Autodesk Inventor part; units mm, degrees
ref_plane "Work Plane1" through (-26.5, -2, 0) normal (-1, 0, 0) x (0, 0, 1)
ref_plane "YZ Plane" through (0, 0, 0) normal (1, 0, 0) x (0, 1, 0)
ref_plane "XZ Plane" through (0, 0, 0) normal (0, 1, 0) x (-1, 0, 0)
sketch "Sketch1" plane through (0, 0, 0) normal (0, 0, 1) x (1, 0, 0)
  line L0 (-25.25, 2.5) -> (25.25, 2.5)
  line L1 (25.25, 2.5) -> (25.25, -2.5)
  line L2 (25.25, -2.5) -> (-25.25, -2.5)
  line L3 (-25.25, -2.5) -> (-25.25, 2.5)
  circle A0 centre (-22.5, 1.3) radius 0.5
  circle A1 centre (-19.4, 1.3) radius 0.4
  circle A2 centre (-10.4, 1.3) radius 0.4
  circle A3 centre (-18, 1.3) radius 0.4
  circle A4 centre (-13.5, 1.3) radius 0.4
  circle A5 centre (-16.6, 1.3) radius 0.4
  circle A6 centre (-14.9, 1.3) radius 0.4
  circle A7 centre (-12.1, 1.3) radius 0.4
  circle A8 centre (-7.6, 1.3) radius 0.4
  circle A9 centre (-9, 1.3) radius 0.4
  line L4 (0, 0) -> (0, 2.997) construction
  line L5 (0, 0) -> (1.9732, 0) construction
  circle A10 centre (-4.5, 1.3) radius 0.5
  circle A11 centre (-1.5, 1.3) radius 0.4
  circle A12 centre (0, 1.3) radius 0.4
  circle A13 centre (1.5, 1.3) radius 0.4
  circle A14 centre (3, 1.3) radius 0.4
  circle A15 centre (4.5, 1.3) radius 0.4
  circle A16 centre (6, 1.3) radius 0.4
  circle A17 centre (7.5, 1.3) radius 0.4
  circle A18 centre (9, 1.3) radius 0.4
  circle A19 centre (10.5, 1.3) radius 0.4
  circle A20 centre (12, 1.3) radius 0.4
  circle A21 centre (13.5, 1.3) radius 0.4
  circle A22 centre (15, 1.3) radius 0.4
  circle A23 centre (18, 1.3) radius 0.625
  circle A24 centre (22.5, 1.3) radius 0.625
  line L6 (-22, 1.3) -> (-22, 2.5)
  line L7 (-23, 1.3) -> (-23, 2.5)
  line L8 (-19, 1.3) -> (-19, 2.5)
  line L9 (-19.8, 1.3) -> (-19.8, 2.5)
  line L10 (-17.6, 1.3) -> (-17.6, 2.5)
  line L11 (-18.4, 1.3) -> (-18.4, 2.5)
  line L12 (-16.2, 1.3) -> (-16.2, 2.5)
  line L13 (-17, 1.3) -> (-17, 2.5)
  line L14 (-14.5, 1.3) -> (-14.5, 2.5)
  line L15 (-15.3, 1.3) -> (-15.3, 2.5)
  line L16 (-13.1, 1.3) -> (-13.1, 2.5)
  line L17 (-13.9, 1.3) -> (-13.9, 2.5)
  line L18 (-11.7, 1.3) -> (-11.7, 2.5)
  line L19 (-12.5, 1.3) -> (-12.5, 2.5)
  line L20 (-10, 1.3) -> (-10, 2.5)
  line L21 (-10.8, 1.3) -> (-10.8, 2.5)
  line L22 (-8.6, 1.3) -> (-8.6, 2.5)
  line L23 (-9.4, 1.3) -> (-9.4, 2.5)
  line L24 (-7.2, 1.3) -> (-7.2, 2.5)
  line L25 (-8, 1.3) -> (-8, 2.5)
  line L26 (-4, 1.3) -> (-4, 2.5)
  line L27 (-5, 1.3) -> (-5, 2.5)
  line L28 (-1.1, 1.3) -> (-1.1, 2.5)
  line L29 (-1.9, 1.3) -> (-1.9, 2.5)
  line L30 (0.4, 1.3) -> (0.4, 2.5)
  line L31 (-0.4, 1.3) -> (-0.4, 2.5)
  line L32 (1.9, 1.3) -> (1.9, 2.5)
  line L33 (1.1, 1.3) -> (1.1, 2.5)
  line L34 (2.6, 1.3) -> (2.6, 2.5)
  line L35 (3.4, 1.3) -> (3.4, 2.5)
  line L36 (4.1, 1.3) -> (4.1, 2.5)
  line L37 (4.9, 1.3) -> (4.9, 2.5)
  line L38 (5.6, 1.3) -> (5.6, 2.5)
  line L39 (6.4, 1.3) -> (6.4, 2.5)
  line L40 (7.1, 1.3) -> (7.1, 2.5)
  line L41 (7.9, 1.3) -> (7.9, 2.5)
  line L42 (8.6, 1.3) -> (8.6, 2.5)
  line L43 (9.4, 1.3) -> (9.4, 2.5)
  line L44 (10.1, 1.3) -> (10.1, 2.5)
  line L45 (10.9, 1.3) -> (10.9, 2.5)
  line L46 (11.6, 1.3) -> (11.6, 2.5)
  line L47 (12.4, 1.3) -> (12.4, 2.5)
  line L48 (13.1, 1.3) -> (13.1, 2.5)
  line L49 (13.9, 1.3) -> (13.9, 2.5)
  line L50 (14.6, 1.3) -> (14.6, 2.5)
  line L51 (15.4, 1.3) -> (15.4, 2.5)
  line L52 (17.375, 1.3) -> (17.375, 2.5)
  line L53 (18.625, 1.3) -> (18.625, 2.5)
  line L54 (23.125, 1.3) -> (23.125, 2.5)
  line L55 (21.875, 1.3) -> (21.875, 2.5)
  circle A25 centre (22.5, -1.3) radius 0.625
  circle A26 centre (18, -1.3) radius 0.625
  circle A27 centre (15, -1.3) radius 0.4
  circle A28 centre (13.5, -1.3) radius 0.4
  circle A29 centre (12, -1.3) radius 0.4
  circle A30 centre (10.5, -1.3) radius 0.4
  circle A31 centre (9, -1.3) radius 0.4
  circle A32 centre (7.5, -1.3) radius 0.4
  circle A33 centre (6, -1.3) radius 0.4
  circle A34 centre (4.5, -1.3) radius 0.4
  circle A35 centre (3, -1.3) radius 0.4
  circle A36 centre (1.5, -1.3) radius 0.4
  circle A37 centre (0, -1.3) radius 0.4
  circle A38 centre (-1.5, -1.3) radius 0.4
  circle A39 centre (-7.5, -1.3) radius 0.4
  circle A40 centre (-9, -1.3) radius 0.4
  circle A41 centre (-10.5, -1.3) radius 0.4
  circle A42 centre (-12.6, -1.3) radius 0.4
  circle A43 centre (-14.4, -1.3) radius 0.4
  circle A44 centre (-16.5, -1.3) radius 0.4
  circle A45 centre (-18, -1.3) radius 0.4
  circle A46 centre (-19.5, -1.3) radius 0.4
  circle A47 centre (-21.6, -1.3) radius 0.4
  circle A48 centre (-23.4, -1.3) radius 0.4
  line L56 (23.125, -1.3) -> (23.125, -2.5)
  line L57 (21.875, -1.3) -> (21.875, -2.5)
  line L58 (18.625, -1.3) -> (18.625, -2.5)
  line L59 (17.375, -1.3) -> (17.375, -2.5)
  line L60 (15.4, -1.3) -> (15.4, -2.5)
  line L61 (14.6, -1.3) -> (14.6, -2.5)
  line L62 (13.9, -1.3) -> (13.9, -2.5)
  line L63 (13.1, -1.3) -> (13.1, -2.5)
  line L64 (12.4, -1.3) -> (12.4, -2.5)
  line L65 (11.6, -1.3) -> (11.6, -2.5)
  line L66 (10.9, -1.3) -> (10.9, -2.5)
  line L67 (10.1, -1.3) -> (10.1, -2.5)
  line L68 (9.4, -1.3) -> (9.4, -2.5)
  line L69 (8.6, -1.3) -> (8.6, -2.5)
  line L70 (7.9, -1.3) -> (7.9, -2.5)
  line L71 (7.1, -1.3) -> (7.1, -2.5)
  line L72 (6.4, -1.3) -> (6.4, -2.5)
  line L73 (5.6, -1.3) -> (5.6, -2.5)
  line L74 (4.9, -1.3) -> (4.9, -2.5)
  line L75 (4.1, -1.3) -> (4.1, -2.5)
  line L76 (3.4, -1.3) -> (3.4, -2.5)
  line L77 (2.6, -1.3) -> (2.6, -2.5)
  line L78 (1.9, -1.3) -> (1.9, -2.5)
  line L79 (1.1, -1.3) -> (1.1, -2.5)
  line L80 (0.4, -1.3) -> (0.4, -2.5)
  line L81 (-0.4, -1.3) -> (-0.4, -2.5)
  line L82 (-1.9, -1.3) -> (-1.9, -2.5)
  line L83 (-1.1, -1.3) -> (-1.1, -2.5)
  line L84 (-7.9, -1.3) -> (-7.9, -2.5)
  line L85 (-7.1, -1.3) -> (-7.1, -2.5)
  line L86 (-8.6, -1.3) -> (-8.6, -2.5)
  line L87 (-9.4, -1.3) -> (-9.4, -2.5)
  line L88 (-10.1, -1.3) -> (-10.1, -2.5)
  line L89 (-10.9, -1.3) -> (-10.9, -2.5)
  line L90 (-12.2, -1.3) -> (-12.2, -2.5)
  line L91 (-13, -1.3) -> (-13, -2.5)
  line L92 (-14, -1.3) -> (-14, -2.5)
  line L93 (-14.8, -1.3) -> (-14.8, -2.5)
  line L94 (-16.1, -1.3) -> (-16.1, -2.5)
  line L95 (-16.9, -1.3) -> (-16.9, -2.5)
  line L96 (-17.6, -1.3) -> (-17.6, -2.5)
  line L97 (-18.4, -1.3) -> (-18.4, -2.5)
  line L98 (-19.1, -1.3) -> (-19.1, -2.5)
  line L99 (-19.9, -1.3) -> (-19.9, -2.5)
  line L100 (-21.2, -1.3) -> (-21.2, -2.5)
  line L101 (-22, -1.3) -> (-22, -2.5)
  line L102 (-23, -1.3) -> (-23, -2.5)
  line L103 (-23.8, -1.3) -> (-23.8, -2.5)
  dimension "d0" = 50.5
  dimension "d1" = 5
  dimension "d3" = 1
  dimension "d4" = 2.75
  dimension "d5" = 0.8
  dimension "d6" = 0.8
  dimension "d7" = 0.8
  dimension "d8" = 0.8
  dimension "d9" = 0.8
  dimension "d10" = 0.8
  dimension "d11" = 0.8
  dimension "d12" = 0.8
  dimension "d13" = 0.8
  dimension "d14" = 3.1
  dimension "d15" = 1.4
  dimension "d16" = 1.4
  dimension "d17" = 1.4
  dimension "d18" = 1.4
  dimension "d19" = 1.7
  dimension "d20" = 1.4
  dimension "d21" = 1.4
  dimension "d22" = 1.7
  dimension "d23" = 1.2
  dimension "d24" = 1
  dimension "d25" = 3.1
  dimension "d26" = 0.8
  dimension "d27" = 0.8
  dimension "d28" = 0.8
  dimension "d29" = 0.8
  dimension "d30" = 0.8
  dimension "d31" = 0.8
  dimension "d32" = 0.8
  dimension "d33" = 0.8
  dimension "d34" = 0.8
  dimension "d35" = 0.8
  dimension "d36" = 0.8
  dimension "d37" = 0.8
  dimension "d38" = 3
  dimension "d39" = 1.5
  dimension "d40" = 1.5
  dimension "d41" = 1.5
  dimension "d42" = 1.5
  dimension "d43" = 1.5
  dimension "d44" = 1.5
  dimension "d45" = 1.5
  dimension "d46" = 1.5
  dimension "d47" = 1.5
  dimension "d48" = 1.5
  dimension "d49" = 1.5
  dimension "d50" = 1.25
  dimension "d51" = 1.25
  dimension "d52" = 3
  dimension "d53" = 4.5
  dimension "d121" = 1.25
  dimension "d122" = 1.25
  dimension "d125" = 0.8
  dimension "d126" = 0.8
  dimension "d127" = 0.8
  dimension "d128" = 0.8
  dimension "d129" = 0.8
  dimension "d130" = 0.8
  dimension "d131" = 0.8
  dimension "d132" = 0.8
  dimension "d133" = 0.8
extrude "Extrusion1" add sketch "Sketch1" along normal blind 2 contours L0 L7 A0 L6 L9 A1 L8 L11 A3 L10 L13 A5 L12 L15 A6 L14 L17 A4 L16 L19 A7 L18 L21 A2 L20 L23 A9 L22 L25 A8 L24 L27 A10 L26 L29 A11 L28 L31 A12 L30 L33 A13 L32 L34 A14 L35 L36 A15 L37 L38 A16 L39 L40 A17 L41 L42 A18 L43 L44 A19 L45 L46 A20 L47 L48 A21 L49 L50 A22 L51 L52 A23 L53 L55 A24 L54 L1 L2 L56 A25 L57 L58 A26 L59 L60 A27 L61 L62 A28 L63 L64 A29 L65 L66 A30 L67 L68 A31 L69 L70 A32 L71 L72 A33 L73 L74 A34 L75 L76 A35 L77 L78 A36 L79 L80 A37 L81 L83 A38 L82 L85 A39 L84 L86 A40 L87 L88 A41 L89 L90 A42 L91 L92 A43 L93 L94 A44 L95 L96 A45 L97 L98 A46 L99 L100 A47 L101 L102 A48 L103 L3
ref_plane "Work Plane1" through (-26.5, -2, 0) normal (-1, 0, 0) x (0, 0, 1)
sketch "Sketch12" plane through (0, 0, 0) normal (0, 0, -1) x (-1, 0, 0)
  arc A0 (-24.0126, -0.5173) -> (-23.9919, 1.0846) centre (-25.2704, 0.3) ccw
  arc A1 (-24.2504, 2) -> (-23.9919, 1.0846) centre (-22.5004, 2) ccw
  arc A2 (-24.0126, -0.5173) -> (-24.2331, -2) centre (-22.5004, -1.5) ccw
  line L0 (-24.2331, -2) -> (-25.0004, -2)
  line L1 (-25.0004, 2) -> (-24.2504, 2)
  line L2 (-25.0004, -2.1) -> (-24.0947, -2.1)
  arc A3 (-23.9286, -0.5716) -> (-23.8794, -2.5) centre (-22.5004, -1.5) ccw
  arc A4 (-23.9286, -0.5716) -> (-23.9067, 1.1369) centre (-25.2704, 0.3) ccw
  arc A5 (-24.1474, 2.1) -> (-23.9067, 1.1369) centre (-22.5004, 2) ccw
  line L3 (-24.1474, 2.1) -> (-25, 2.1)
  line L4 (-24.1474, 2.1) -> (-24.1474, 2.5)
  line L5 (-25.25, 2.5) -> (-23.125, 2.5)
  line L6 (-24.1474, 2.5) -> (-25.25, 2.5)
  line L7 (-23.125, -2.5) -> (-25.25, -2.5)
  line L8 (-25.25, 2.5) -> (-25.25, -2.5)
  line L9 (-25.25, -2.5) -> (-24.0947, -2.5)
  line L10 (-24.0947, -2.1) -> (-24.0947, -2.5)
  point P0 (0, 0)
  dimension "d188" = 0.1
extrude "Extrusion12" cut sketch "Sketch12" against normal blind 10
sketch "Sketch13" plane through (0, 0, 0) normal (0, 0, -1) x (-1, 0, 0)
  arc A0 (24.3834, 0.9639) -> (24.3834, -0.9639) centre (26.1358, 0) ccw
  arc A1 (24.3834, 0.9639) -> (24.6496, 2) centre (22.4996, 2) ccw
  arc A2 (24.6496, -2) -> (24.3834, -0.9639) centre (22.4996, -2) ccw
  line L0 (24.6496, -2) -> (25, -2)
  line L1 (24.9996, 2) -> (24.6496, 2)
  line L2 (24.6496, 2) -> (24.6496, 2.5)
  line L3 (23, 2.5) -> (25.25, 2.5)
  line L4 (24.6496, -2) -> (24.6496, -2.5)
  line L5 (25.25, -2.5) -> (23.8, -2.5)
  line L6 (24.6496, -2.5) -> (25.25, -2.5)
  line L7 (25.25, -2.5) -> (25.25, 2.5)
  line L8 (25.25, 2.5) -> (25.25, -2.5)
  line L9 (25.25, 2.5) -> (24.6496, 2.5)
  line L10 (25, -2.1) -> (24.5471, -2.1)
  arc A3 (24.5471, -2.1) -> (24.2958, -1.012) centre (22.4996, -2) ccw
  arc A4 (24.2958, 1.012) -> (24.2958, -1.012) centre (26.1358, 0) ccw
  arc A5 (24.2958, 1.012) -> (24.5471, 2.1) centre (22.4996, 2) ccw
  line L11 (24.5471, 2.1) -> (25, 2.1)
  line L12 (24.55, -2.6) -> (25.35, -2.6)
  line L13 (25.35, -2.6) -> (25.35, 2.6)
  line L14 (25.35, 2.6) -> (24.55, 2.6)
  line L15 (24.5471, -2.5) -> (24.6496, -2.5)
  line L16 (24.6496, 2.5) -> (24.5471, 2.5)
  line L17 (24.5471, 2.1) -> (24.5471, 2.5)
  line L18 (24.5471, 2.5) -> (24.6496, 2.5)
  line L19 (24.5471, -2.1) -> (24.5471, -2.5)
  line L20 (24.5471, -2.5) -> (24.6496, -2.5)
  point P0 (0, 0)
  dimension "d193" = 0.1
extrude "Extrusion13" cut sketch "Sketch13" against normal blind 10
sketch "Sketch14" plane through (0, 0, 0) normal (0, 0, -1) x (-1, 0, 0)
  arc A0 (6.3296, -2) -> (4.9596, -2) centre (5.6446, -2) ccw
  arc A1 (4.9596, -2) -> (6.3296, -2) centre (5.6446, -2) ccw
  arc A2 (4.0396, -2) -> (2.6696, -2) centre (3.3546, -2) ccw
  arc A3 (2.6696, -2) -> (4.0396, -2) centre (3.3546, -2) ccw
  arc A4 (4.1396, -2) -> (2.5696, -2) centre (3.3546, -2) ccw
  arc A5 (2.5696, -2) -> (4.1396, -2) centre (3.3546, -2) ccw
  arc A6 (6.4296, -2) -> (4.8596, -2) centre (5.6446, -2) ccw
  arc A7 (4.8596, -2) -> (6.4296, -2) centre (5.6446, -2) ccw
  point P0 (0, 0)
  dimension "d195" = 0.1
  dimension "d196" = 0.1
extrude "Extrusion14" cut sketch "Sketch14" against normal blind 10 contours A1 A0 | A3 A2 | A5 A4 | A7 A6
sketch "Sketch15" plane through (0, 0, 2) normal (0, 0, 1) x (1, 0, 0)
  line L0 (-23.8, -0.675) -> (23.125, -0.675)
  line L1 (23.125, -0.675) -> (23.125, -2.5)
  line L2 (23.125, -2.5) -> (-23.8, -2.5)
  line L3 (-23.8, -2.5) -> (-23.8, -0.675)
  line L4 (-23.8, -2.5) -> (-23.8, -1.3)
  line L5 (23.125, -1.3) -> (23.125, -2.5)
  line L6 (18.625, -2.5) -> (21.875, -2.5)
  arc A0 (23.125, -1.3) -> (21.875, -1.3) centre (22.5, -1.3) ccw
  line L7 (-24.5471, -2.5) -> (-23.8, -2.5)
  line L8 (-24.5496, 2.5) -> (-23.8, 2.5)
  line L9 (-23.8, 2.5) -> (-23.8, -2.5)
  line L10 (-23.8, -2.5) -> (-24.5496, -2.5)
  line L11 (24.2038, 2.5) -> (23.125, 2.5)
  line L12 (23.125, 2.5) -> (23.125, -2.5)
  line L13 (23.125, -2.5) -> (24.2038, -2.5)
  arc A1 (23.8794, -2.5) -> (23.9286, -0.5716) centre (22.5004, -1.5) ccw
  line L14 (-24.5496, 2.5117) -> (-24.5496, -2.5071)
  arc A2 (-24.2958, -1.012) -> (-24.5471, -2.1) centre (-22.4996, -2) ccw
  line L15 (24.2038, -2.5071) -> (24.2038, 2.5117)
  point P0 (0, 0)
  point P1 (-23.8, -1.9)
  point P2 (23.125, -1.9)
  point P3 (20.25, -2.5)
  point P4 (22.5, -0.675)
  point P5 (24.1474, 2.5)
extrude "Extrusion15" add sketch "Sketch15" against normal up to surface (2 mm away)
properties part number "3d_LM-Welding_Tooling - Top Comb" material "Steel, Carbon"
Geometry: final body of the model. Coordinates: model frame, mm. Coordinates: 2 decimals unless noted, no trailing zeros. Loops run counter-clockwise (first coordinate to the right, second up) from the corner with the lowest first, then second, coordinate; pieces in that order, holes last. Notation, with made-up numbers: (-18.5, 75) -> (1.5, 75) arc R5 ccw to (1.5, 80) -> close; hole circle Ø8 at (32.25, -1.75). An arc over 180 degrees is marked (long way). Use a Markdown table: item, result. Add a question column.
(1) Section query A-A, the plane x = 4.5. Return loops of the section in (y, z).
(2) Section query B-B, the plane y = 1.9. State how many separate pieces and enclosed holes the cut face has, plus the area to 3 significant figures.
(3) Line query: line 1 along Y through (x, z) = (-18, 1.9). Output: solid intervals per line, ascending.
(4) Mould query, pull axis X, two halves, no side actions, for faces 1 (the flat face through (4.9, 2, 1)), 2 (the flat face through (0, -2.5, 1)). Classes: pulls with the +X half, pulls with the -X half, needs draft (parallel to the pull), parting line crosses it, or undercut.
(5) Section query C-C, the plane x = 18. Return loops of the section in (y, z) (3 decimals), plus the area to 3 significant figures.
Answer:
| question | item | result |
|---|---|---|
| 1 | outline | (-2.5, 0) -> (0.9, 0) -> (0.9, 2) -> (-2.5, 2) -> close |
| 2 | separate pieces | 26 |
| 2 | enclosed holes | 0 |
| 2 | area | 54.9 mm^2 |
| 3 | line 1 | y = -2.5 to 0.9 |
| 4 | face 1 | undercut |
| 4 | face 2 | needs draft |
| 5 | outline | (-2.5, 0) -> (0.675, 0) -> (0.675, 2) -> (-2.5, 2) -> close |
| 5 | area | 6.35 mm^2 |
